Here's how the part is built. I have some questions about the finished solid (model axes, mm). Give positions to 0.01 mm unless a question says otherwise; leave off trailing zeros. Loops run counter-clockwise (first coordinate to the right, second up) from the corner with the lowest first, then second, coordinate; pieces in that order, holes last.
Q1. Will this pin go through, and if not, where does the flat tip stop? P1, Ø5, axis at x = -25.5, y = -14, coming from the +Z side.
Q2. I need wall thicknesses on line 1 (X direction, y = -2, z = 1.75); line 2 (Y direction, x = 16.5, z = 2.25); line 3 (X direction, y = -1, z = 3.5). Which ranges of each line are inside material? Lowest first, please.
Q3. If we section it at C-C (x = 19.5): Please give me the cut outline in (y, z), plus the area to 3 significant figures.
Q4. If we section it at B-B (y = -3): Please give me the cut outline in (x, z).
Q5. If we section it at A-A (x = -4): Please give me the cut outline in (y, z).
Q6. If we section it at D-D (y = 15): Please give me the cut outline in (x, z).
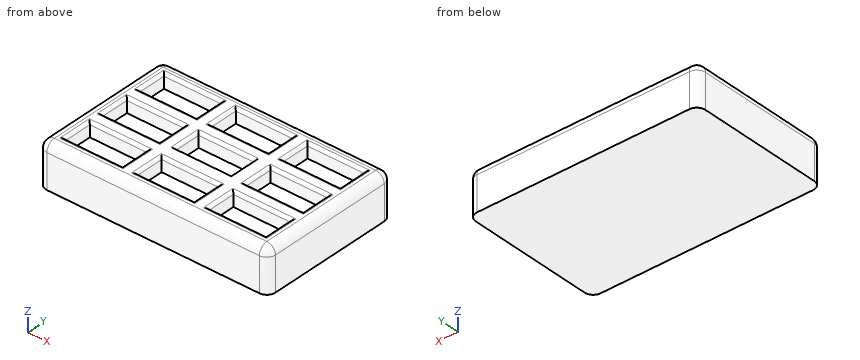
from build123d import *

# Parameters (mm, degrees)
F0_W     = 80
F0_H     = 50
F0_W_2   = 20
F0_H_2   = 10
F1_DEPTH = 10
F2_DEPTH = 5
F3_R     = 3
F4_R     = 1


with BuildPart() as f1:
    # F0 (on Top) → F1 (new body)
    with BuildSketch(Plane.XY):
        Rectangle(F0_W, F0_H)
        with Locations((-25, -15)):
            Rectangle(F0_W_2, F0_H_2, mode=Mode.SUBTRACT)
        with Locations((0, -15)):
            Rectangle(F0_W_2, F0_H_2, mode=Mode.SUBTRACT)
        with Locations((25, -15)):
            Rectangle(F0_W_2, F0_H_2, mode=Mode.SUBTRACT)
        with Locations((-25, 0)):
            Rectangle(F0_W_2, F0_H_2, mode=Mode.SUBTRACT)
        with Locations((-25, 15)):
            Rectangle(F0_W_2, F0_H_2, mode=Mode.SUBTRACT)
        Rectangle(F0_W_2, F0_H_2, mode=Mode.SUBTRACT)
        with Locations((25, 0)):
            Rectangle(F0_W_2, F0_H_2, mode=Mode.SUBTRACT)
        with Locations((0, 15)):
            Rectangle(F0_W_2, F0_H_2, mode=Mode.SUBTRACT)
        with Locations((25, 15)):
            Rectangle(F0_W_2, F0_H_2, mode=Mode.SUBTRACT)
        with Locations((-25, 15)):
            Rectangle(F0_W_2, F0_H_2)
        with Locations((0, 15)):
            Rectangle(F0_W_2, F0_H_2)
        with Locations((25, 15)):
            Rectangle(F0_W_2, F0_H_2)
        with Locations((25, 0)):
            Rectangle(F0_W_2, F0_H_2)
        Rectangle(F0_W_2, F0_H_2)
        with Locations((-25, 0)):
            Rectangle(F0_W_2, F0_H_2)
        with Locations((-25, -15)):
            Rectangle(F0_W_2, F0_H_2)
        with Locations((0, -15)):
            Rectangle(F0_W_2, F0_H_2)
        with Locations((25, -15)):
            Rectangle(F0_W_2, F0_H_2)
    extrude(amount=-F1_DEPTH)

    # F0 (on Top) → F2 (join)
    with BuildSketch(Plane.XY):
        Rectangle(F0_W, F0_H)
        with Locations((-25, -15)):
            Rectangle(F0_W_2, F0_H_2, mode=Mode.SUBTRACT)
        with Locations((0, -15)):
            Rectangle(F0_W_2, F0_H_2, mode=Mode.SUBTRACT)
        with Locations((25, -15)):
            Rectangle(F0_W_2, F0_H_2, mode=Mode.SUBTRACT)
        with Locations((-25, 0)):
            Rectangle(F0_W_2, F0_H_2, mode=Mode.SUBTRACT)
        with Locations((-25, 15)):
            Rectangle(F0_W_2, F0_H_2, mode=Mode.SUBTRACT)
        Rectangle(F0_W_2, F0_H_2, mode=Mode.SUBTRACT)
        with Locations((25, 0)):
            Rectangle(F0_W_2, F0_H_2, mode=Mode.SUBTRACT)
        with Locations((0, 15)):
            Rectangle(F0_W_2, F0_H_2, mode=Mode.SUBTRACT)
        with Locations((25, 15)):
            Rectangle(F0_W_2, F0_H_2, mode=Mode.SUBTRACT)
    extrude(amount=F2_DEPTH)

    # F3
    f3_edges = [f1.edges().sort_by_distance(p)[0] for p in [
        (-40, -25, -2.5),
        (40, -25, -2.5),
        (0, -25, 5),
        (-40, 0, 5),
        (40, 0, 5),
        (40, 25, -2.5),
        (0, 25, 5),
        (-40, 25, -2.5),
    ]]
    fillet(f3_edges, radius=F3_R)

    # F4
    f4_edges = [f1.edges().sort_by_distance(p)[0] for p in [
        (-15, -15, 5),
        (-25, -10, 5),
        (-35, -15, 5),
        (-25, -20, 5),
        (-15, 0, 5),
        (-25, -5, 5),
        (-35, 0, 5),
        (-25, 5, 5),
        (-25, 20, 5),
        (-15, 15, 5),
        (-25, 10, 5),
        (-35, 15, 5),
        (-10, 15, 5),
        (0, 20, 5),
        (0, 10, 5),
        (10, 15, 5),
        (0, 5, 5),
        (-10, 0, 5),
        (-10, -15, 5),
        (0, -10, 5),
        (0, -20, 5),
        (10, -15, 5),
        (15, 0, 5),
        (25, 5, 5),
        (15, 15, 5),
        (25, 20, 5),
        (25, -5, 5),
        (15, -15, 5),
        (25, -10, 5),
        (25, -20, 5),
        (35, -15, 5),
        (35, 0, 5),
        (35, 15, 5),
        (25, 10, 5),
    ]]
    fillet(f4_edges, radius=F4_R)


solid = f1.part
Check sheet entries:
1. P1: stops at z = 0
2. line 1: x = -40 to -35, -15 to -10, 10 to 15, 35 to 40
2. line 2: y = -24.99 to -20, -10 to -5, 5 to 10, 20 to 24.99
2. line 3: x = -39.6 to -35, -15 to -10, 10 to 15, 35 to 39.6
3. outline: (-25, -10) - (25, -10) - (25, 2) arc R3 ccw to (22, 5) - (21, 5) arc R1 ccw to (20, 4) - (20, 0) - (10, 0) - (10, 4) arc R1 ccw to (9, 5) - (6, 5) arc R1 ccw to (5, 4) - (5, 0) - (-5, 0) - (-5, 4) arc R1 ccw to (-6, 5) - (-9, 5) arc R1 ccw to (-10, 4) - (-10, 0) - (-20, 0) - (-20, 4) arc R1 ccw to (-21, 5) - (-22, 5) arc R3 ccw to (-25, 2) - close
3. area: 595 mm2
4. outline: (-40, -10) - (40, -10) - (40, 2) arc R3 ccw to (37, 5) - (36, 5) arc R1 ccw to (35, 4) - (35, 0) - (15, 0) - (15, 4) arc R1 ccw to (14, 5) - (10, 5) - (10, 0) - (-10, 0) - (-10, 4) arc R1 ccw to (-11, 5) - (-14, 5) arc R1 ccw to (-15, 4) - (-15, 0) - (-35, 0) - (-35, 4) arc R1 ccw to (-36, 5) - (-37, 5) arc R3 ccw to (-40, 2) - close
5. outline: (-25, -10) - (25, -10) - (25, 2) arc R3 ccw to (22, 5) - (21, 5) arc R1 ccw to (20, 4) - (20, 0) - (10, 0) - (10, 4) arc R1 ccw to (9, 5) - (6, 5) arc R1 ccw to (5, 4) - (5, 0) - (-5, 0) - (-5, 5) - (-9, 5) arc R1 ccw to (-10, 4) - (-10, 0) - (-20, 0) - (-20, 4) arc R1 ccw to (-21, 5) - (-22, 5) arc R3 ccw to (-25, 2) - close
6. outline: (-40, -10) - (40, -10) - (40, 2) arc R3 ccw to (37, 5) - (36, 5) arc R1 ccw to (35, 4) - (35, 0) - (15, 0) - (15, 4) arc R1 ccw to (14, 5) - (11, 5) arc R1 ccw to (10, 4) - (10, 0) - (-10, 0) - (-10, 4) arc R1 ccw to (-11, 5) - (-14, 5) arc R1 ccw to (-15, 4) - (-15, 0) - (-35, 0) - (-35, 4) arc R1 ccw to (-36, 5) - (-37, 5) arc R3 ccw to (-40, 2) - close
